Answer from the drawing. Dimensions are ordinates in mm from the lowest x, y and z of the part. Give positions to 0.01 mm unless a question says otherwise; leave off trailing zeros. Write each loop counter-clockwise with the first axis right and the second up, starting at its lowest first coordinate (ties: lowest second). Pieces come first, ordered by that corner, then holes. Notation, with made-up numbers: M 3.25,10 L 23.25,10 A25 ccw 23.25,28 Z; hole C 83,27.5 d8. An arc over 180 degrees is marked long. Answer as a JSON object with one key per item and string values.
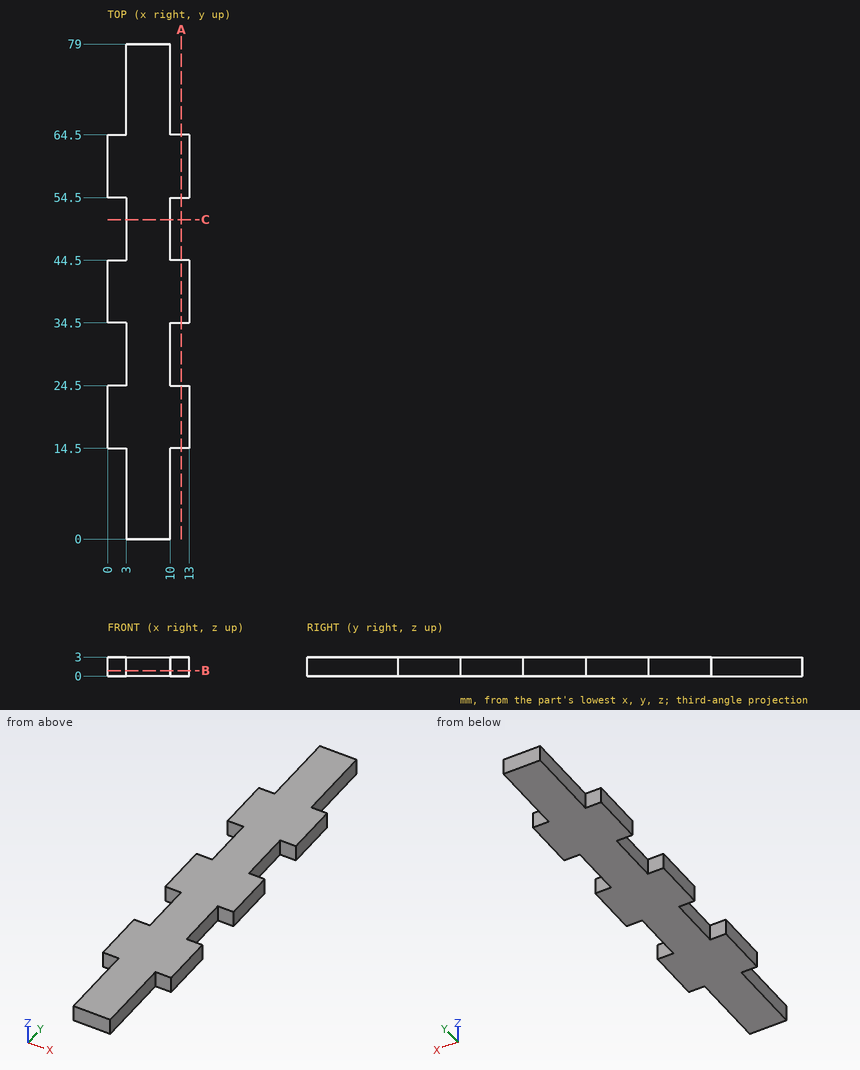
1. Consider line 1 along Y through (x, z) = (2, 0.6); line 2 along X through (y, z) = (47.5, 2.7). Determine where each line is inside the solid, lowest interval first.
Verdict:
{"line 1": "y = 14.5 to 24.5, 34.5 to 44.5, 54.5 to 64.5", "line 2": "x = 3 to 10"}
2. A cutting plane is placed at C-C, the plane y = 51. Give the vertices of the cut face in (x, z), plus the area to 3 significant figures.
Verdict:
{"outline": "M 3,0 L 10,0 L 10,3 L 3,3 Z", "area": "21.0 mm2"}
3. Flat-ended cylindrical pins translate along their axes: pin 1 (1.5 mm diameter, centred on x = 1, z = 2, fed in from +Y); pin 2 (0.9 mm diameter, centred on x = 1, z = 2, fed in from -Y); pin 3 (1.5 mm diameter, centred on y = 7.5, z = 2, fed in from -X). Find the tip coordinate at first contact, or state that the pin passes through.
Verdict:
{"pin 1": "stops at y = 64.5", "pin 2": "stops at y = 14.5", "pin 3": "stops at x = 3"}
4. A cutting plane is placed at A-A, the plane x = 11.75. Give the vertices of the cut face in (y, z), plus the area to 3 significant figures.
Verdict:
{"outline": "M 14.5,0 L 24.5,0 L 24.5,3 L 14.5,3 Z; M 34.5,0 L 44.5,0 L 44.5,3 L 34.5,3 Z; M 54.5,0 L 64.5,0 L 64.5,3 L 54.5,3 Z", "area": "90.0 mm2"}
5. A cutting plane is placed at B-B, the plane z = 0.85. Give the vertices of the cut face in (x, y), plus the area to 3 significant figures.
Verdict:
{"outline": "M 0,14.5 L 3,14.5 L 3,0 L 10,0 L 10,14.5 L 13,14.5 L 13,24.5 L 10,24.5 L 10,34.5 L 13,34.5 L 13,44.5 L 10,44.5 L 10,54.5 L 13,54.5 L 13,64.5 L 10,64.5 L 10,79 L 3,79 L 3,64.5 L 0,64.5 L 0,54.5 L 3,54.5 L 3,44.5 L 0,44.5 L 0,34.5 L 3,34.5 L 3,24.5 L 0,24.5 Z", "area": "733 mm2"}
